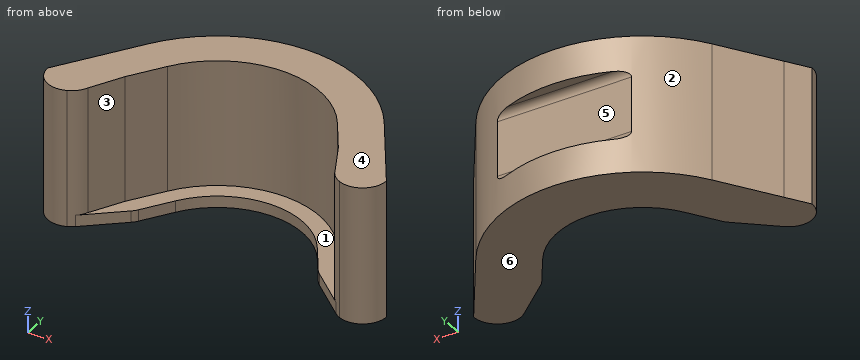
```python
from build123d import *

# Parameters (mm, degrees)
F1_DEPTH    = 12
F2_W        = 1.5
F2_H        = 6
F3_DEPTH    = 12.5
F4_R        = 0.6
F5_T1_DEPTH = 12
F7_DEPTH    = 1


# Not quite as in the source:
# - a fillet or chamfer that OpenCascade refuses, or shapes differently, is made with other operations: its cross-section is extruded or revolved along the edge and cut away or added


with BuildPart() as f1:
    # F0 (on Top) → F1 (new body)
    with BuildSketch(Plane.XY):
        with BuildLine():
            ThreePointArc((-7.5164818898, 24.95), (0, 29), (7.5164818898, 24.95))
            Line((7.5164818898, 24.95), (10.7763181216, 20))
            Line((10.7763181216, 20), (14.9671085022, 20))
            Line((14.9671085022, 20), (10.4395581803, 26.875))
            ThreePointArc((10.4395581803, 26.875), (0, 32.5), (-10.4395581803, 26.875))
            Line((-10.4395581803, 26.875), (-13.6993944121, 21.925))
            ThreePointArc((-13.6993944121, 21.925), (-11.7192459572, 21.75), (-10.7763181216, 20))
            Line((-10.7763181216, 20), (-7.5164818898, 24.95))
        make_face()
        with BuildLine():
            Line((14.9671085022, 20), (10.7763181216, 20))
            Line((10.7763181216, 20), (12.0440322117, 18.075))
            ThreePointArc((12.0440322117, 18.075), (14.0241806666, 18.25), (14.9671085022, 20))
        make_face()
        with BuildLine():
            Line((12.0440322117, 18.075), (10.7763181216, 20))
            ThreePointArc((10.7763181216, 20), (11.1217133119, 18.8475326453), (12.0440322117, 18.075))
        make_face()
        with BuildLine():
            ThreePointArc((-12.0440322117, 18.075), (-11.1217133119, 18.8475326453), (-10.7763181216, 20))
            Line((-10.7763181216, 20), (-12.0440322117, 18.075))
        make_face()
        with BuildLine():
            Line((-12.0440322117, 18.075), (-10.7763181216, 20))
            Line((-10.7763181216, 20), (-14.9671085022, 20))
            ThreePointArc((-14.9671085022, 20), (-14.0241806666, 18.25), (-12.0440322117, 18.075))
        make_face()
        with BuildLine():
            Line((-14.9671085022, 20), (-10.7763181216, 20))
            ThreePointArc((-10.7763181216, 20), (-11.7192459572, 21.75), (-13.6993944121, 21.925))
            Line((-13.6993944121, 21.925), (-14.9671085022, 20))
        make_face()
    extrude(amount=F1_DEPTH)

    # F2 (on Right) → F3 (cut, symmetric)
    with BuildSketch(Plane.YZ):
        with Locations((31.75, 6)):
            Rectangle(F2_W, F2_H)
    extrude(amount=F3_DEPTH, both=True, mode=Mode.SUBTRACT)

    # F4
    f4_edges = [f1.edges().sort_by_distance(p)[0] for p in [
        (0, 31, 9),
        (0, 31, 3),
    ]]
    fillet(f4_edges, radius=F4_R)

    # F5: chamfer of 5 on 2 edges, made by hand

    # F5_s2 → F5_t1 (join)
    with BuildSketch(Plane.XY):
        with BuildLine():
            Line((11.0273555293, 19.0260146009), (9.3449019992, 22.2084505142))
            Line((9.3449019992, 22.2084505142), (9.4284184646, 22.2634505142))
            ThreePointArc((9.4284184646, 22.2634505142), (10.1361174506, 21.1539508584), (10.859834587, 20.055))
            Line((10.859834587, 20.055), (10.8763181216, 20))
            ThreePointArc((10.8763181216, 20), (10.9346351532, 19.5211157003), (11.1198360632, 19.0640586655))
            Line((11.1198360632, 19.0640586655), (11.0273555293, 19.0260146009))
        make_face()
        with BuildLine():
            Line((-9.3449019992, 22.2084505142), (-11.0273555293, 19.0260146009))
            Line((-11.0273555293, 19.0260146009), (-11.1198360632, 19.0640586655))
            ThreePointArc((-11.1198360632, 19.0640586655), (-10.9346351532, 19.5211157003), (-10.8763181216, 20))
            Line((-10.8763181216, 20), (-10.859834587, 20.055))
            ThreePointArc((-10.859834587, 20.055), (-10.1361174506, 21.1539508584), (-9.4284184646, 22.2634505142))
            Line((-9.4284184646, 22.2634505142), (-9.3449019992, 22.2084505142))
        make_face()
    extrude(amount=F5_T1_DEPTH)

    # F6 (on face) → F7 (join)
    with BuildSketch(Plane(origin=(0, 0, 0), x_dir=(1, 0, 0), z_dir=(0, 0, -1))):
        with BuildLine():
            ThreePointArc((-7.5164818898, -24.95), (0, -29), (7.5164818898, -24.95))
            Line((7.5164818898, -24.95), (9.4383768754, -22.0316386155))
            Line((9.4383768756, -22.0316386152), (10.9338806529, -19.2028264998))
            ThreePointArc((10.9338806529, -19.2028264998), (11.1736784475, -18.772254667), (11.507412541, -18.4096024365))
            Line((11.507412541, -18.4096024365), (8.3196064123, -21.1442182701))
            ThreePointArc((8.3196064123, -21.1442182701), (8.1209139726, -21.3403362232), (7.9514665684, -21.5622112204))
            Line((7.9514665684, -21.5622112204), (6.2637349082, -24.125))
            ThreePointArc((6.2637349082, -24.125), (0, -27.5), (-6.2637349082, -24.125))
            Line((-6.2637349082, -24.125), (-7.9514665684, -21.5622112204))
            ThreePointArc((-7.9514665684, -21.5622112204), (-8.1209139726, -21.3403362232), (-8.3196064123, -21.1442182701))
            Line((-8.3196064123, -21.1442182701), (-11.507412541, -18.4096024365))
            ThreePointArc((-11.507412541, -18.4096024365), (-11.1736784475, -18.772254667), (-10.9338806529, -19.2028264998))
            Line((-10.9338806529, -19.2028264998), (-9.4383768756, -22.0316386152))
            Line((-9.4383768756, -22.0316386152), (-7.5164818898, -24.95))
        make_face()
    extrude(amount=-F7_DEPTH)


solid = f1.part
```
CAD build for the part. Positions are in the model's coordinates, mm. Face numbers are marked on the shaded views. A direction names the side the tool comes from. Round coordinates to 2 decimals unless told otherwise and drop trailing zeros. Order: outer loops, then holes, each group sorted by start corner. A loop starts at its lowest first (then second) coordinate and runs counter-clockwise, first axis right, second up. Notation, with made-up numbers: (78, 68.25) - (96, 68.25) arc R25 cw to (96, 105.25) - close; hole circle Ø9 at (57, -26). An arc over 180 degrees is marked (long way). Use CSV: the item, a comma, the result in double quotes. Start each with the question number.
1) Wall check: L1, parallel to Z at x = -6.5, y = 25.25; L2, parallel to X at y = 25.5, z = 10.5; L3, parallel to X at y = 24.5, z = 6.5. Give the ranges that are in metal, low to high. Write a range as [from, to].
2) Tool access for the marked faces 1 and 2: list every direction of +Z, -Z, +X, -X, +Y, -Y with a clear straight run to the whole face (end or side of a thin tool).
3) Saw through at C-C (x = 3.5). List the corners of the cut face in (y, z).
4) Saw through at A-A (y = 23). List the corners of the cut face in (x, z).
5) Saw through at B-B (z = 4.5). List the corners of the cut face in (x, y) (3 decimals), and give its area (3 significant figures).
6) Saw through at D-D (y = 26). List the corners of the cut face in (x, z), and give its area (3 significant figures).
7) Two-plate mould, pull along Z, no slides. Class the marked faces 3, 4, 5 and 6: pulls with the +Z half, pulls with the -Z half, needs draft (parallel to the pull), parting line crosses it, or undercut.
8) Pin check, flat tips, straight feed: pin 1 Ø6 at (x, z) = (6.5, 9) entering from -Y; pin 2 Ø3 at (x, y) = (-7, 20.5) entering from -Z; pin 3 Ø4 at (x, z) = (-3, 6) entering from +Y; pin 4 Ø3 at (y, z) = (22.5, 10.5) entering from +X. Stop position of each tip, or through.
Values follow:
1,L1,"z = [0, 1]"
1,L2,"x = [-11.35, -7.12], [7.12, 11.35]"
1,L3,"x = [-12, -7.81], [7.81, 12]"
2,face 1,"+Z, -Y"
2,face 2,"+Z, -Z, +Y"
3,outline,"(26.63, 0) - (32, 0) - (32, 3) - (31.6, 3) arc R0.6 cw to (31, 3.6) - (31, 8.4) arc R0.6 cw to (31.6, 9) - (32, 9) - (32, 12) - (28.29, 12) - (28.29, 1) - (26.63, 1) - close"
4,outline,"(-12.99, 0) - (-7, 0) - (-7, 1) - (-8.8, 1) - (-8.8, 12) - (-12.99, 12) - close; (7, 0) - (12.99, 0) - (12.99, 12) - (8.8, 12) - (8.8, 1) - (7, 1) - close"
5,outline,"(-14.967, 20) arc R2.095 ccw to (-10.934, 19.203) - (-9.438, 22.032) - (-7.516, 24.95) arc R9 cw to (7.516, 24.95) - (9.438, 22.032) - (10.934, 19.203) arc R2.095 ccw to (14.967, 20) - (10.44, 26.875) arc R12.5 ccw to (5.937, 31) - (-5.937, 31) arc R12.5 ccw to (-10.44, 26.875) - close"
5,area,"126 mm2"
6,outline,"(-11.02, 0) - (-4.5, 0) - (-4.5, 1) - (-6.71, 1) - (-6.71, 12) - (-11.02, 12) - close; (4.5, 0) - (11.02, 0) - (11.02, 12) - (6.71, 12) - (6.71, 1) - (4.5, 1) - close"
6,area,"108 mm2"
7,face 3,"needs draft"
7,face 4,"pulls with the +Z half"
7,face 5,"undercut"
7,face 6,"pulls with the -Z half"
8,pin 1,"stops at y = 21.92"
8,pin 2,"stops at z = 0"
8,pin 3,"stops at y = 31"
8,pin 4,"stops at x = 14.31"
